Here's how the part is built. I have some questions about the finished solid (model axes, mm). A direction names the side the tool comes from. Round coordinates to 2 decimals unless told otherwise and drop trailing zeros. Loops run counter-clockwise (first coordinate to the right, second up) from the corner with the lowest first, then second, coordinate; pieces in that order, holes last. Notation, with made-up numbers: M 52.25,59.25 L 96.25,59.25 A11 ccw 96.25,72.25 Z; hole C -28.75,88.25 d6. An arc over 180 degrees is marked long. Answer as CSV lines item,"result".
```python
from build123d import *

# Parameters (mm, degrees)
F0_R     = 60
F3_DEPTH = 5
F1_R     = 24
F2_W     = 80
F2_H     = 80
F4_DEPTH = 5.001
F5_R     = 5
F6_R     = 5


with BuildPart() as f3:
    # F0 (on Top) → F3 (new body)
    with BuildSketch(Plane.XY):
        Circle(F0_R)
    extrude(amount=-F3_DEPTH)

    # F1 (on Top) + F2 (on Top) → F4 (cut, through all)
    with BuildSketch(Plane.XY):
        with Locations((0, 30)):
            Circle(F1_R)
    with BuildSketch(Plane.XY):
        with Locations((0, -50)):
            Rectangle(F2_W, F2_H)
    extrude(amount=-F4_DEPTH, mode=Mode.SUBTRACT)

    # F5
    f5_edges = [f3.edges().sort_by_distance(p)[0] for p in [
        (-40, -10, -2.5),
        (40, -10, -2.5),
    ]]
    fillet(f5_edges, radius=F5_R)

    # F6
    f6_edges = [f3.edges().sort_by_distance(p)[0] for p in [
        (-40, -44.72136, -2.5),
        (40, -44.72136, -2.5),
    ]]
    fillet(f6_edges, radius=F6_R)


solid = f3.part
```
1. For P1, Ø1.5, axis at y = -4.5, z = -1, coming from the +X side; P2, Ø2, axis at y = 10.5, z = -4, coming from the -X side; P3, Ø1, axis at y = -18.5, z = -2, coming from the -X side; P4, Ø6, axis at x = 41.5, y = 20.5, coming from the +Z side, each with a flat end and sliding along its axis, tell me the tip position at first contact or that it passes through.
Evaluation:
P1,"stops at x = 59.88"
P2,"stops at x = -59.24"
P3,"stops at x = -57.24"
P4,"stops at z = 0"
2. I want a section at B-B, the plane y = 42.5. Please give me the cut outline in (x, z), and give its area (3 significant figures).
Evaluation:
outline,"M -42.35,-5 L -20.49,-5 L -20.49,0 L -42.35,0 Z; M 20.49,-5 L 42.35,-5 L 42.35,0 L 20.49,0 Z"
area,"219 mm²"
3. We'd pull the mould along X, two halves only. Please class faces 1 (the flat face through (-40, -23, -2)), 2 (the flat face through (40, -23, -2)), 3 (the cylindrical face through (1.834, 59.972, -2.465)), 4 (the flat face through (-1, 2, -5)): pulls with the +X half, pulls with the -X half, needs draft (parallel to the pull), parting line crosses it, or undercut.
Evaluation:
face 1,"undercut"
face 2,"undercut"
face 3,"parting line crosses it"
face 4,"needs draft"
4. I want a section at C-C, the plane z = -0.85. Please give me the cut outline in (x, y).
Evaluation:
outline,"M -49.09,-34.5 A5 ccw -40,-31.62 L -40,-15 A5 cw -35,-10 L 35,-10 A5 cw 40,-15 L 40,-31.62 A5 ccw 49.09,-34.5 A60 ccw long Z; hole C 0,30 d48"
5. If I drill on line 1 (Y direction, x = 0, z = -3.65); line 2 (X direction, y = 29.5, z = -3.1); line 3 (X direction, y = 35, z = -1.9), over which ranges is the centre line in solid material (lowest first)? Write a range as [from, to].
Evaluation:
line 1,"y = [-10, 6], [54, 60]"
line 2,"x = [-52.25, -23.99], [23.99, 52.25]"
line 3,"x = [-48.73, -23.47], [23.47, 48.73]"
6. Which directions (+Z, -Z, +X, -X, +Y, -Y) give clear straight access to the entire face, cutting with the end or side of a thin tool? Please do faces 5 (the cylindrical face through (-23.977, 31.055, -2.465)), 6 (the flat face through (0, -10, -2)).
Evaluation:
face 5,"+Z, -Z"
face 6,"+Z, -Z, -Y"
7. I want a section at D-D, the plane x = 42. Please give me the cut outline in (y, z).
Evaluation:
outline,"M -35.62,-5 L 42.85,-5 L 42.85,0 L -35.62,0 Z"
8. I want a section at A-A, the plane x = 0. Please give me the cut outline in (y, z).
Evaluation:
outline,"M -10,-5 L 6,-5 L 6,0 L -10,0 Z; M 54,-5 L 60,-5 L 60,0 L 54,0 Z"
